Input: part model. Units: mm. Frame: model coordinates. Face numbers are marked on the shaded views. Coordinates: 2 decimals unless noted, no trailing zeros.
Autodesk Inventor part; units mm, degrees
ref_plane "YZ Plane" through (0, 0, 0) normal (1, 0, 0) x (0, 1, 0)
ref_plane "XZ Plane" through (0, 0, 0) normal (0, 1, 0) x (-1, 0, 0)
ref_plane "XY Plane" through (0, 0, 0) normal (0, 0, 1) x (1, 0, 0)
sketch "スケッチ1" plane through (0, 0, 0) normal (0, 1, 0) x (-1, 0, 0)
  circle A0 centre (0, 0) radius 55
  dimension "d0" = 110
extrude "押し出し1" add sketch "スケッチ1" along normal blind 2.2
sketch "スケッチ2" plane through (0, 2.2, 0) normal (0, 1, 0) x (1, 0, 0)
  circle A0 centre (0, 0) radius 62.5
  line L0 (-4.8484, -32.3614) -> (6.4919, -32.3614) construction
  line L1 (6.4919, -32.3614) -> (6.4919, -37.029) construction
  line L2 (6.4919, -37.029) -> (-4.8484, -37.029) construction
  line L3 (-4.8484, -37.029) -> (-4.8484, -32.3614) construction
  dimension "d3" = 125
extrude "押し出し2" add sketch "スケッチ2" along normal blind 3.4
chamfer "面取り1" distance 0.75 angle 45 1 edges at (-62.5, 2.2, 0)
chamfer "面取り2" distance 0.75 angle 45 1 edges at (-62.5, 5.6, 0)
sketch "スケッチ3" plane through (0, 0, 0) normal (0, -1, 0) x (1, 0, 0)
  circle A0 centre (0, 0) radius 62.5
  dimension "d12" = 125
extrude "押し出し3" add sketch "スケッチ3" along normal blind 3.4
chamfer "面取り3" distance 0.75 angle 45 1 edges at (-62.5, 0, 0)
chamfer "面取り4" distance 0.75 angle 45 1 edges at (-62.5, -3.4, 0)
sketch "スケッチ6" plane through (0, 5.6, 0) normal (0, 1, 0) x (1, 0, 0)
  circle A0 centre (0, 0) radius 7.65
  line L0 (0, 7.65) -> (46.8799, 7.65)
  circle A1 centre (0, 0) radius 47.5
  line L1 (0, -7.65) -> (46.8799, -7.65)
  dimension "d39" = 15.3
extrude "押し出し5" [suppressed]
chamfer "面取り7" [suppressed]
chamfer "面取り8" [suppressed]
chamfer "面取り9" [suppressed]
sketch "スケッチ7" plane through (0, 5.6, 0) normal (0, 1, 0) x (1, 0, 0)
  line L0 (-9.3358, -20.9354) -> (21.308, -20.9354) construction
  line L1 (21.308, -20.9354) -> (21.308, -27.5341) construction
  line L2 (21.308, -27.5341) -> (-9.3358, -27.5341) construction
  line L3 (-9.3358, -27.5341) -> (-9.3358, -20.9354) construction
  spline S0 degree 2 poles (-5.7914, -21.6571) (-5.2131, -21.667) (-4.2541, -22.0526) (-3.9377, -22.3739) knots 0 0 0 1 2 2 2
  spline S1 degree 2 poles (-3.9377, -22.3739) (-3.646, -22.6754) (-3.3247, -23.5207) (-3.3247, -24.0645) knots 0 0 0 1 2 2 2
  spline S2 degree 2 poles (-3.3247, -24.0645) (-3.3247, -24.633) (-3.6708, -25.5079) (-3.9772, -25.8045) knots 0 0 0 1 2 2 2
  spline S3 degree 2 poles (-3.9772, -25.8045) (-4.3084, -26.1308) (-5.2773, -26.4916) (-5.7914, -26.5015) knots 0 0 0 1 2 2 2
  line L4 (-5.7914, -26.5015) -> (-5.7914, -27.2084)
  line L5 (-5.7914, -27.2084) -> (-6.6021, -27.2084)
  line L6 (-6.6021, -27.2084) -> (-6.6021, -26.5015)
  spline S4 degree 2 poles (-6.6021, -26.5015) (-7.1162, -26.4867) (-8.0802, -26.1506) (-8.4213, -25.8144) knots 0 0 0 1 2 2 2
  spline S5 degree 2 poles (-8.4213, -25.8144) (-8.7277, -25.5129) (-9.0688, -24.628) (-9.0688, -24.0645) knots 0 0 0 1 2 2 2
  spline S6 degree 2 poles (-9.0688, -24.0645) (-9.0688, -23.5306) (-8.7426, -22.6853) (-8.446, -22.3788) knots 0 0 0 1 2 2 2
  spline S7 degree 2 poles (-8.446, -22.3788) (-8.1296, -22.0526) (-7.1805, -21.672) (-6.6021, -21.6571) knots 0 0 0 1 2 2 2
  line L7 (-6.6021, -21.6571) -> (-6.6021, -21.0096)
  line L8 (-6.6021, -21.0096) -> (-5.7914, -21.0096)
  line L9 (-5.7914, -21.0096) -> (-5.7914, -21.6571)
  spline S8 degree 2 poles (-5.7914, -25.8886) (-5.4207, -25.8787) (-4.8473, -25.6562) (-4.6594, -25.4684) knots 0 0 0 1 2 2 2
  spline S9 degree 2 poles (-4.6594, -25.4684) (-4.4073, -25.2212) (-4.17, -24.5143) (-4.17, -24.0299) knots 0 0 0 1 2 2 2
  spline S10 degree 2 poles (-4.17, -24.0299) (-4.17, -23.6245) (-4.3974, -22.9572) (-4.6248, -22.7249) knots 0 0 0 1 2 2 2
  spline S11 degree 2 poles (-4.6248, -22.7249) (-4.8374, -22.5024) (-5.4009, -22.2899) (-5.7914, -22.28) knots 0 0 0 1 2 2 2
  line L10 (-5.7914, -22.28) -> (-5.7914, -25.8886)
  spline S12 degree 2 poles (-6.6021, -22.28) (-6.9926, -22.2849) (-7.5562, -22.5074) (-7.7687, -22.7249) knots 0 0 0 1 2 2 2
  spline S13 degree 2 poles (-7.7687, -22.7249) (-7.9961, -22.9523) (-8.2235, -23.6344) (-8.2235, -24.0299) knots 0 0 0 1 2 2 2
  spline S14 degree 2 poles (-8.2235, -24.0299) (-8.2235, -24.5143) (-7.9862, -25.2262) (-7.7341, -25.4684) knots 0 0 0 1 2 2 2
  spline S15 degree 2 poles (-7.7341, -25.4684) (-7.5463, -25.6463) (-6.9729, -25.8836) (-6.6021, -25.8886) knots 0 0 0 1 2 2 2
  line L11 (-6.6021, -25.8886) -> (-6.6021, -22.28)
  line L12 (0.8424, -27.159) -> (-2.1334, -27.159)
  line L13 (-2.1334, -27.159) -> (-2.1334, -26.5361)
  line L14 (-2.1334, -26.5361) -> (-1.0261, -26.5361)
  line L15 (-1.0261, -26.5361) -> (-1.0261, -22.448)
  line L16 (-1.0261, -22.448) -> (-2.1334, -22.448)
  line L17 (-2.1334, -22.448) -> (-2.1334, -21.8895)
  spline S16 degree 2 poles (-2.1334, -21.8895) (-1.5056, -21.8895) (-0.9124, -21.5335) (-0.8729, -21.0392) knots 0 0 0 1 2 2 2
  line L18 (-0.8729, -21.0392) -> (-0.2401, -21.0392)
  line L19 (-0.2401, -21.0392) -> (-0.2401, -26.5361)
  line L20 (-0.2401, -26.5361) -> (0.8424, -26.5361)
  line L21 (0.8424, -26.5361) -> (0.8424, -27.159)
  line L22 (5.4199, -27.159) -> (2.4441, -27.159)
  line L23 (2.4441, -27.159) -> (2.4441, -26.5361)
  line L24 (2.4441, -26.5361) -> (3.5514, -26.5361)
  line L25 (3.5514, -26.5361) -> (3.5514, -22.448)
  line L26 (3.5514, -22.448) -> (2.4441, -22.448)
  line L27 (2.4441, -22.448) -> (2.4441, -21.8895)
  spline S17 degree 2 poles (2.4441, -21.8895) (3.0719, -21.8895) (3.6651, -21.5335) (3.7046, -21.0392) knots 0 0 0 1 2 2 2
  line L28 (3.7046, -21.0392) -> (4.3373, -21.0392)
  line L29 (4.3373, -21.0392) -> (4.3373, -26.5361)
  line L30 (4.3373, -26.5361) -> (5.4199, -26.5361)
  line L31 (5.4199, -26.5361) -> (5.4199, -27.159)
  spline S18 degree 2 poles (10.3385, -24.109) (10.3385, -25.7502) (9.3844, -27.2875) (8.3908, -27.2875) knots 0 0 0 1 2 2 2
  spline S19 degree 2 poles (8.3908, -27.2875) (7.3824, -27.2875) (6.4382, -25.7205) (6.4382, -24.1139) knots 0 0 0 1 2 2 2
  spline S20 degree 2 poles (6.4382, -24.1139) (6.4382, -22.4629) (7.3923, -20.9354) (8.3908, -20.9354) knots 0 0 0 1 2 2 2
  spline S21 degree 2 poles (8.3908, -20.9354) (9.3943, -20.9354) (10.3385, -22.5173) (10.3385, -24.109) knots 0 0 0 1 2 2 2
  spline S22 degree 2 poles (9.2905, -25.9677) (9.4091, -25.6661) (9.508, -24.7368) (9.508, -24.109) knots 0 0 0 1 2 2 2
  spline S23 degree 2 poles (9.508, -24.109) (9.508, -23.4812) (9.4091, -22.5568) (9.2856, -22.2454) knots 0 0 0 1 2 2 2
  spline S24 degree 2 poles (9.2856, -22.2454) (9.162, -21.9339) (8.7319, -21.6126) (8.3908, -21.6126) knots 0 0 0 1 2 2 2
  spline S25 degree 2 poles (8.3908, -21.6126) (8.0497, -21.6126) (7.6098, -21.9339) (7.4813, -22.2553) knots 0 0 0 1 2 2 2
  spline S26 degree 2 poles (7.4813, -22.2553) (7.3577, -22.5667) (7.2687, -23.5158) (7.2687, -24.1139) knots 0 0 0 1 2 2 2
  spline S27 degree 2 poles (7.2687, -24.1139) (7.2687, -24.7566) (7.3478, -25.6167) (7.4763, -25.9528) knots 0 0 0 1 2 2 2
  spline S28 degree 2 poles (7.4763, -25.9528) (7.595, -26.2692) (8.0349, -26.6103) (8.3908, -26.6103) knots 0 0 0 1 2 2 2
  spline S29 degree 2 poles (8.3908, -26.6103) (8.727, -26.6103) (9.1669, -26.289) (9.2905, -25.9677) knots 0 0 0 1 2 2 2
  point P0 (0, 0)
extrude "押し出し6" add sketch "スケッチ7" along normal blind 0.5
sketch "スケッチ8" plane through (0, 5.6, 0) normal (0, 1, 0) x (1, 0, 0)
  line L0 (-53, 6) -> (-59, 6)
  line L1 (-59, 6) -> (-59, -6)
  line L2 (-59, -6) -> (-53, -6)
  line L3 (-53, -6) -> (-53, 6)
  circle A0 centre (0, 0) radius 55
  point P0 (-56, -6)
  point P1 (-56, 6)
  point P2 (-55, 0)
  point P3 (-55, 0)
  dimension "d53" = 12
  dimension "d54" = 6
  dimension "d55" = 53
extrude "押し出し7" cut sketch "スケッチ8" against normal blind 10 contours L3 L2 A0 L0 | A0 L2 L1 L0 picked at (-53.6545, -0.6678)
sketch "スケッチ9" plane through (0, 5.6, 0) normal (0, 1, 0) x (1, 0, 0)
  point P0 (0, 0)
  point P1 (0, 0)
hole "穴2" at (0, 5.6, 0) direction (0, -1, 0) diameter 15.5 end through all
sketch "スケッチ10" plane through (0, 5.6, 0) normal (0, 1, 0) x (1, 0, 0)
  circle A0 centre (0, 0) radius 12.5 construction
  point P0 (0, -12.5)
  point P1 (12.5, 0)
  point P2 (0, 12.5)
  point P3 (-12.5, 0)
  dimension "d67" = 25
  dimension "d81" = 360
hole "穴3" at (0, 5.6, 12.5) at (-12.5, 5.6, 0) at (0, 5.6, -12.5) at (12.5, 5.6, 0) direction (0, -1, 0) diameter 3.2 end through all
properties part number "pully_shoulder2_110"
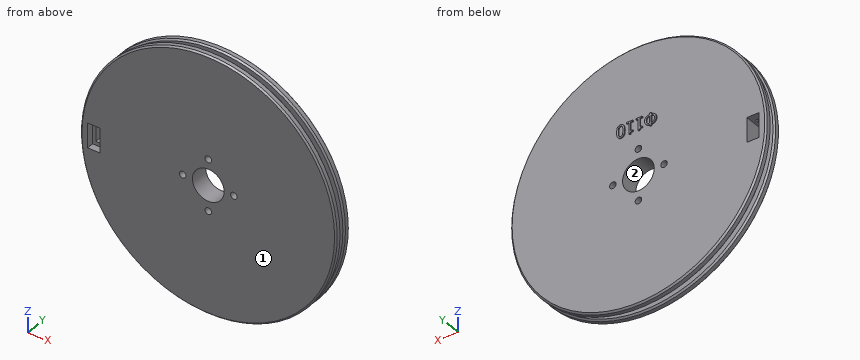
Item 1: Pin query (flat end, axial travel): pin 1 Ø1.5 at (y, z) = (4, -12) entering from -X; pin 2 Ø1 at (y, z) = (3.5, -29.5) entering from -X; pin 3 Ø5 at (x, y) = (14.5, 4.5) entering from +Z. Return the tip coordinate at first contact, or that it passes through.
Response values:
pin 1: stops at x = -61.48
pin 2: stops at x = -55.36
pin 3: stops at z = 61.34
Item 2: Draft query along X for the marked faces 1 and 2. Return one class per face: pulls with the +X half, pulls with the -X half, needs draft (parallel to the pull), parting line crosses it, or undercut.
Response values:
face 1: needs draft
face 2: undercut
Item 3: Ray query, probe 1 along X at (y, z) = (0.5, 0); probe 2 along X at (y, z) = (3.5, 0); probe 3 along Y at (x, z) = (-39, -40). Return the intervals inside material, ascending.
Response values:
probe 1: x = -53 to -14.1, -10.9 to -7.75, 7.75 to 10.9, 14.1 to 55
probe 2: x = -62.5 to -59, -53 to -14.1, -10.9 to -7.75, 7.75 to 10.9, 14.1 to 62.5
probe 3: y = -3.4 to 0, 2.2 to 5.6
Item 4: Cut plane A-A on z = 0. Count the separate pieces of the cut face and the enclosed holes in it, then the cut area to 3 significant figures.
Response values:
separate pieces: 6
enclosed holes: 0
area: 847 mm2
